```python
from build123d import *

# Parameters (mm, degrees)
F0_W     = 304.8
F0_H     = 127
F0_W_2   = 136.525
F0_H_2   = 114.3
F1_DEPTH = 3.175
F2_W     = 12.7
F2_H     = 25.4
F3_DEPTH = 25.4
F5_D     = 6.7564


with BuildPart() as f1:
    # F0 (on Top) → F1 (new body)
    with BuildSketch(Plane.XY):
        with Locations((152.4, 63.5)):
            Rectangle(F0_W, F0_H)
        with Locations((80.9625, 63.5)):
            Rectangle(F0_W_2, F0_H_2, mode=Mode.SUBTRACT)
        with Locations((223.8375, 63.5)):
            Rectangle(F0_W_2, F0_H_2, mode=Mode.SUBTRACT)
    extrude(amount=F1_DEPTH)

    # F2 (on face) → F3 (join)
    with BuildSketch(Plane(origin=(0, 0, 0), x_dir=(1, 0, 0), z_dir=(0, 0, -1))):
        with Locations((6.35, -63.5)):
            Rectangle(F2_W, F2_H)
        with Locations((298.45, -63.5)):
            Rectangle(F2_W, F2_H)
    extrude(amount=F3_DEPTH)

    # F5 (through all)
    with Locations(Plane(origin=(0, 0, -25.4), x_dir=(1, 0, 0), z_dir=(0, 0, -1))):
        with Locations((6.35, -63.5), (298.45, -63.5)):
            Hole(F5_D / 2)


solid = f1.part
```
Design review of the part built by this model. Coordinates are the model's own, in mm. A direction names the side the tool comes from. Round coordinates to 2 decimals unless told otherwise and drop trailing zeros. Write each loop counter-clockwise with the first axis right and the second up, starting at its lowest first coordinate (ties: lowest second). Pieces come first, ordered by that corner, then holes. Notation, with made-up numbers: (57, -17) -> (95, -17) arc R22 ccw to (95, -11) -> close; hole circle Ø9 at (35.5, 34). An arc over 180 degrees is marked (long way). Answer in a Markdown table with one row per item.
Q1. Draft analysis for pull direction X (two halves, no side actions). For faces 5 (the face through (12.7, 63, -9)), 6 (the face through (6, 76.2, -13)), 7 (the face through (0, 63, -7)), state which applies: +X half, -X half, draft (parallel to the pull), parting line (faces both ways), or undercut.
The answers:
| item | result |
|---|---|
| face 5 | undercut |
| face 6 | draft |
| face 7 | -X half |
Q2. For faces 1 (the face through (292.1, 63, -9)), 2 (the face through (298, 50.8, -13)), 3 (the face through (298, 76.2, -13)), 4 (the face through (304.8, 63, -7)), list the 3-axis set-ups (+Z, -Z, +X, -X, +Y, -Y) from which the entire face can be reached by the end or side of a thin tool; tool diameter is ignored.
The answers:
| item | result |
|---|---|
| face 1 | +Z, -Z |
| face 2 | -Z, +X, -X, -Y |
| face 3 | -Z, +X, -X, +Y |
| face 4 | +Z, -Z, +X, +Y, -Y |
Q3. Take a section at C-C, the plane x = 298.45. State the section outline as (y, z) points (3 decimals).
The answers:
| item | result |
|---|---|
| outline | (0, 0) -> (50.8, 0) -> (50.8, -25.4) -> (60.122, -25.4) -> (60.122, 3.175) -> (0, 3.175) -> close; (66.878, -25.4) -> (76.2, -25.4) -> (76.2, 0) -> (127, 0) -> (127, 3.175) -> (66.878, 3.175) -> close |
Q4. Take a section at B-B, the plane y = 63.5. State the section outline as (x, z) points (3 decimals).
The answers:
| item | result |
|---|---|
| outline | (0, -25.4) -> (2.972, -25.4) -> (2.972, 3.175) -> (0, 3.175) -> close; (9.728, -25.4) -> (12.7, -25.4) -> (12.7, 3.175) -> (9.728, 3.175) -> close; (149.225, 0) -> (155.575, 0) -> (155.575, 3.175) -> (149.225, 3.175) -> close; (292.1, -25.4) -> (295.072, -25.4) -> (295.072, 3.175) -> (292.1, 3.175) -> close; (301.828, -25.4) -> (304.8, -25.4) -> (304.8, 3.175) -> (301.828, 3.175) -> close |
Q5. Clearance check with flat-ended pins moving along their axes: pin 1 Ø10 at (x, z) = (6.5, -11) entering from -Y; pin 2 Ø6.5 at (x, z) = (7.5, -14) entering from +Y; pin 3 Ø3.5 at (y, z) = (71.5, 2) entering from -X. State where each tip first meets the part, or that it passes through.
The answers:
| item | result |
|---|---|
| pin 1 | y = 50.8 |
| pin 2 | y = 76.2 |
| pin 3 | x = 0 |
Q6. Take a section at A-A, the plane z = -16.75. State the section outline as (x, y) points.
The answers:
| item | result |
|---|---|
| outline | (0, 50.8) -> (12.7, 50.8) -> (12.7, 76.2) -> (0, 76.2) -> close; (292.1, 50.8) -> (304.8, 50.8) -> (304.8, 76.2) -> (292.1, 76.2) -> close; hole circle Ø6.76 at (6.35, 63.5); hole circle Ø6.76 at (298.45, 63.5) |
Q7. Take a section at D-D, the plane y = 22. State the section outline as (x, z) points (3 decimals), then the cut area to 3 significant figures.
The answers:
| item | result |
|---|---|
| outline | (0, 0) -> (12.7, 0) -> (12.7, 3.175) -> (0, 3.175) -> close; (149.225, 0) -> (155.575, 0) -> (155.575, 3.175) -> (149.225, 3.175) -> close; (292.1, 0) -> (304.8, 0) -> (304.8, 3.175) -> (292.1, 3.175) -> close |
| area | 101 mm² |
Q8. To check wall thickness, follow L1, parallel to X at y = 63.5, z = -19.5; L2, parallel to X at y = 36, z = 0.5 (3 decimals); L3, parallel to Y at x = 298.45, z = -16.75. State the ranges of each line that lie inside material, in increasing order. Write a range as [from, to].
The answers:
| item | result |
|---|---|
| L1 | [0, 2.97], [9.73, 12.7], [292.1, 295.07], [301.83, 304.8] |
| L2 | [0, 12.7], [149.225, 155.575], [292.1, 304.8] |
| L3 | [50.8, 60.12], [66.88, 76.2] |
